The listing builds one solid part. Answer for the finished solid, in the listing's coordinates (mm). Round coordinates to 2 decimals unless told otherwise and drop trailing zeros. Write each loop counter-clockwise with the first axis right and the second up, starting at its lowest first coordinate (ties: lowest second). Pieces come first, ordered by that corner, then holes. Notation, with made-up numbers: M 35,81 L 57,81 A25 ccw 57,99 Z; hole C 23.5,80 d8. An arc over 180 degrees is marked long. Write each question's results on one line, items separated by ' | '.
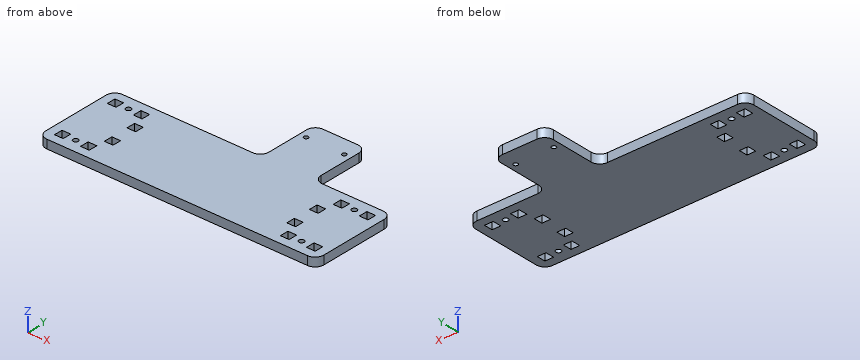
from build123d import *

# Parameters (mm, degrees)
BOSS_EXTRUDE1_OUTLINE_W   = 5
BOSS_EXTRUDE1_OUTLINE_H   = 5
BOSS_EXTRUDE1_OUTLINE_R   = 1.5
BOSS_EXTRUDE1_OUTLINE_R_2 = 1.25
BOSS_EXTRUDE1_DEPTH       = 5
FILLET1_R                 = 5


# Read off the part's stored shape, not the designer's step: Boss-Extrude1
with BuildPart() as part:
    # Boss-Extrude1 outline → Boss-Extrude1 (new body)
    with BuildSketch(Plane.XY):
        Polygon((5, 25), (-80, 25), (-80, -25), (80, -25), (80, 25), (35, 25), (35, 60), (5, 60), align=None)
        with Locations((-72.5, -17.5)):
            Rectangle(BOSS_EXTRUDE1_OUTLINE_W, BOSS_EXTRUDE1_OUTLINE_H, mode=Mode.SUBTRACT)
        with Locations((-65, -17.5)):
            Circle(BOSS_EXTRUDE1_OUTLINE_R, mode=Mode.SUBTRACT)
        with Locations((-57.5, -17.5)):
            Rectangle(BOSS_EXTRUDE1_OUTLINE_W, BOSS_EXTRUDE1_OUTLINE_H, mode=Mode.SUBTRACT)
        with Locations((-52.5, -7.5)):
            Rectangle(BOSS_EXTRUDE1_OUTLINE_W, BOSS_EXTRUDE1_OUTLINE_H, mode=Mode.SUBTRACT)
        with Locations((-52.5, 7.5)):
            Rectangle(BOSS_EXTRUDE1_OUTLINE_W, BOSS_EXTRUDE1_OUTLINE_H, mode=Mode.SUBTRACT)
        with Locations((57.5, -17.5)):
            Rectangle(BOSS_EXTRUDE1_OUTLINE_W, BOSS_EXTRUDE1_OUTLINE_H, mode=Mode.SUBTRACT)
        with Locations((65, -17.5)):
            Circle(BOSS_EXTRUDE1_OUTLINE_R, mode=Mode.SUBTRACT)
        with Locations((72.5, -17.5)):
            Rectangle(BOSS_EXTRUDE1_OUTLINE_W, BOSS_EXTRUDE1_OUTLINE_H, mode=Mode.SUBTRACT)
        with Locations((52.5, -7.5)):
            Rectangle(BOSS_EXTRUDE1_OUTLINE_W, BOSS_EXTRUDE1_OUTLINE_H, mode=Mode.SUBTRACT)
        with Locations((52.5, 7.5)):
            Rectangle(BOSS_EXTRUDE1_OUTLINE_W, BOSS_EXTRUDE1_OUTLINE_H, mode=Mode.SUBTRACT)
        with Locations((-72.5, 17.5)):
            Rectangle(BOSS_EXTRUDE1_OUTLINE_W, BOSS_EXTRUDE1_OUTLINE_H, mode=Mode.SUBTRACT)
        with Locations((-65, 17.5)):
            Circle(BOSS_EXTRUDE1_OUTLINE_R, mode=Mode.SUBTRACT)
        with Locations((-57.5, 17.5)):
            Rectangle(BOSS_EXTRUDE1_OUTLINE_W, BOSS_EXTRUDE1_OUTLINE_H, mode=Mode.SUBTRACT)
        with Locations((57.5, 17.5)):
            Rectangle(BOSS_EXTRUDE1_OUTLINE_W, BOSS_EXTRUDE1_OUTLINE_H, mode=Mode.SUBTRACT)
        with Locations((65, 17.5)):
            Circle(BOSS_EXTRUDE1_OUTLINE_R, mode=Mode.SUBTRACT)
        with Locations((72.5, 17.5)):
            Rectangle(BOSS_EXTRUDE1_OUTLINE_W, BOSS_EXTRUDE1_OUTLINE_H, mode=Mode.SUBTRACT)
        with Locations((9, 50)):
            Circle(BOSS_EXTRUDE1_OUTLINE_R_2, mode=Mode.SUBTRACT)
        with Locations((31, 50)):
            Circle(BOSS_EXTRUDE1_OUTLINE_R_2, mode=Mode.SUBTRACT)
    extrude(amount=BOSS_EXTRUDE1_DEPTH)

    # Fillet1
    fillet1_edges = [part.edges().sort_by_distance(p)[0] for p in [
        (5, 25, 2.5),
        (5, 60, 2.5),
        (35, 60, 2.5),
        (35, 25, 2.5),
        (80, 25, 2.5),
        (80, -25, 2.5),
        (-80, -25, 2.5),
        (-80, 25, 2.5),
    ]]
    fillet(fillet1_edges, radius=FILLET1_R)


solid = part.part
1) Find the intervals of material crossed by line 1 (Y direction, x = -65, z = 2.85); line 2 (Y direction, x = 52.5, z = 0.8); line 3 (X direction, y = -6, z = 3.5), in increasing order.
Return value:
line 1: -25 to -19, -16 to 16, 19 to 25 | line 2: -25 to -10, -5 to 5, 10 to 25 | line 3: -80 to -55, -50 to 50, 55 to 80
2) Section B-B (y = 7.5) is taken. Determine the outline of the cut face in (x, z), then the cut area to 3 significant figures.
Return value:
outline: M -80,0 L -55,0 L -55,5 L -80,5 Z; M -50,0 L 50,0 L 50,5 L -50,5 Z; M 55,0 L 80,0 L 80,5 L 55,5 Z | area: 750 mm²
3) Section A-A (x = -65) is taken. Determine the outline of the cut face in (y, z), then the cut area to 3 significant figures.
Return value:
outline: M -25,0 L -19,0 L -19,5 L -25,5 Z; M -16,0 L 16,0 L 16,5 L -16,5 Z; M 19,0 L 25,0 L 25,5 L 19,5 Z | area: 220 mm²
4) Section D-D (z = 1.75) is taken. State how many separate pieces and enclosed holes the cut face has, then the cut area to 3 significant figures.
Return value:
separate pieces: 1 | enclosed holes: 18 | area: 8,690 mm²
5) This flat-tipped pin is pushed along its axis until it touches: pin 1 (3 mm diameter, centred on x = 47, z = 4.5, fed in from +Y). Where does it stop, or does it pass through?
Return value:
pin 1: y = 25
6) Section C-C (y = 17.5) is taken. Determine the outline of the cut face in (x, z), then the cut area to 3 significant figures.
Return value:
outline: M -80,0 L -75,0 L -75,5 L -80,5 Z; M -70,0 L -66.5,0 L -66.5,5 L -70,5 Z; M -63.5,0 L -60,0 L -60,5 L -63.5,5 Z; M -55,0 L 55,0 L 55,5 L -55,5 Z; M 60,0 L 63.5,0 L 63.5,5 L 60,5 Z; M 66.5,0 L 70,0 L 70,5 L 66.5,5 Z; M 75,0 L 80,0 L 80,5 L 75,5 Z | area: 670 mm²
